Input: part model. Units: mm. Frame: model coordinates. A direction names the side the tool comes from. Coordinates: 2 decimals unless noted, no trailing zeros. Loops run counter-clockwise (first coordinate to the right, second up) from the corner with the lowest first, then second, coordinate; pieces in that order, holes last. Notation, with made-up numbers: (20, -8) -> (73, -8) arc R28 cw to (73, 25) -> close; hole circle Ø7 at (60, -12.5). An arc over 180 degrees is marked (long way). Answer as a JSON object with one key per item and string values.
from build123d import *

# Parameters (mm, degrees)
F0_W     = 146.05
F0_H     = 412.75
F0_H_2   = 406.4
F0_H_3   = 19.05
F1_DEPTH = 19.05


with BuildPart() as f1:
    # F0 (on Right) → F1 (new body)
    with BuildSketch(Plane.YZ):
        with Locations((-73.025, 212.725)):
            Rectangle(F0_W, F0_H)
        with Locations((73.025, 212.725)):
            Rectangle(F0_W, F0_H)
        Polygon((146.05, -12.7), (0, -12.7), (0, -419.1), (82.55, -419.1), (82.55, -381), (146.05, -381), align=None)
        with Locations((-73.025, -215.9)):
            Rectangle(F0_W, F0_H_2)
        with Locations((-73.025, -3.175)):
            Rectangle(F0_W, F0_H_3)
    extrude(amount=F1_DEPTH)


solid = f1.part
1. Section query A-A (y = 93). Return loops of the section in (x, z).
Reply:
{"outline": "(0, -381) -> (19.05, -381) -> (19.05, -12.7) -> (0, -12.7) -> close; (0, 6.35) -> (19.05, 6.35) -> (19.05, 419.1) -> (0, 419.1) -> close"}
2. Access query for faces 1 (the face through (9, 82.55, -400)), 2 (the face through (9, 0, -3)), 3 (the face through (19.05, -2, 6)). Directions: +Z, -Z, +X, -X, +Y, -Y. A direction counts if a zero-diameter tool reaches every point of the face in a straight line with its end or side. Return the directions, or none.
Reply:
{"face 1": "-Z, +X, -X, +Y", "face 2": "+X, -X, +Y", "face 3": "+Z, -Z, +X, +Y, -Y"}
3. Pin query (flat end, axial travel): P1, Ø9.5, axis at x = 10, y = 104.5, coming from the -Z side; P2, Ø9.5, axis at x = 14, z = -1.5, coming from the +Y side; P3, Ø5.5, axis at x = 5, z = -405, coming from the +Y side. Return the tip coordinate at first contact, or that it passes through.
Reply:
{"P1": "stops at z = -381", "P2": "stops at y = 0", "P3": "stops at y = 82.55"}
4. Mould query, pull axis Z, two halves, no side actions, for faces 4 (the face through (0, -2, 6)), 5 (the face through (9, 114, -381)), 6 (the face through (9, 2, 419.1)), 7 (the face through (9, 72, 6.35)). Classes: pulls with the +Z half, pulls with the -Z half, needs draft (parallel to the pull), parting line crosses it, or undercut.
Reply:
{"face 4": "needs draft", "face 5": "pulls with the -Z half", "face 6": "pulls with the +Z half", "face 7": "undercut"}
5. Section query C-C (y = 40). Return loops of the section in (x, z).
Reply:
{"outline": "(0, -419.1) -> (19.05, -419.1) -> (19.05, -12.7) -> (0, -12.7) -> close; (0, 6.35) -> (19.05, 6.35) -> (19.05, 419.1) -> (0, 419.1) -> close"}
6. Section query B-B (x = 8.5). Return loops of the section in (y, z).
Reply:
{"outline": "(-146.05, -419.1) -> (82.55, -419.1) -> (82.55, -381) -> (146.05, -381) -> (146.05, -12.7) -> (0, -12.7) -> (0, 6.35) -> (146.05, 6.35) -> (146.05, 419.1) -> (-146.05, 419.1) -> close"}
7. Line query: line 1 along Z through (x, y) = (7, 11). Output: solid intervals per line, ascending.
Reply:
{"line 1": "z = -419.1 to -12.7, 6.35 to 419.1"}
